from build123d import *

# Parameters (mm, degrees)
F0_W     = 600
F0_H     = 200
F1_DEPTH = 290
F2_R     = 50
F3_T     = -2


with BuildPart() as f1:
    # F0 (on Front) → F1 (new body)
    with BuildSketch(Plane.XZ):
        with Locations((300, 100)):
            Rectangle(F0_W, F0_H)
    extrude(amount=F1_DEPTH)

    # F2
    f2_edges = [f1.edges().sort_by_distance(p)[0] for p in [
        (600, -290, 100),
        (0, -290, 100),
        (600, 0, 100),
        (600, -145, 0),
        (300, -290, 0),
        (0, -145, 0),
        (0, 0, 100),
        (300, 0, 0),
    ]]
    fillet(f2_edges, radius=F2_R)

    # F3
    f3_openings = [f1.faces().sort_by_distance(p)[0] for p in [
        (300, -145, 200),
    ]]
    offset(amount=F3_T, openings=f3_openings)


solid = f1.part
Source: CAD feature listing. Evaluate the final solid. Frame: model axes, mm. A direction names the side the tool comes from. Give positions to 0.01 mm unless a question says otherwise; leave off trailing zeros. Order: outer loops, then holes, each group sorted by start corner. A loop starts at its lowest first (then second) coordinate and runs counter-clockwise, first axis right, second up. Notation, with made-up numbers: (-5, 78.5) -> (33, 78.5) arc R22 ccw to (33, 84.5) -> close; hole circle Ø3 at (35, -23). An arc over 180 degrees is marked (long way). Use a Markdown table: item, result.
1) Contact query for flat-ended pins moving along their axis: P1, Ø5, axis at x = 500.5, y = -116, coming from the +Z side; P2, Ø8, axis at y = -260.5, z = 154, coming from the -X side. Output: stop coordinate, or through.
Answer list:
| item | result |
|---|---|
| P1 | z = 2 |
| P2 | x = 2.8 |
2) Section query C-C, the plane x = 82. Return the cut outline in (y, z), then the cut area to 3 significant figures.
Answer list:
| item | result |
|---|---|
| outline | (-290, 50) arc R50 ccw to (-240, 0) -> (-50, 0) arc R50 ccw to (0, 50) -> (0, 200) -> (-2, 200) -> (-2, 50) arc R48 cw to (-50, 2) -> (-240, 2) arc R48 cw to (-288, 50) -> (-288, 200) -> (-290, 200) -> close |
| area | 1,290 mm² |
3) Section query A-A, the plane z = 114. Return the cut outline in (x, y).
Answer list:
| item | result |
|---|---|
| outline | (0, -240) arc R50 ccw to (50, -290) -> (550, -290) arc R50 ccw to (600, -240) -> (600, -50) arc R50 ccw to (550, 0) -> (50, 0) arc R50 ccw to (0, -50) -> close; hole (2, -240) arc R48 ccw to (50, -288) -> (550, -288) arc R48 ccw to (598, -240) -> (598, -50) arc R48 ccw to (550, -2) -> (50, -2) arc R48 ccw to (2, -50) -> close |
4) Ray query, line 1 along Y through (x, z) = (219.5, 85); line 2 along X through (y, z) = (-61, 99); line 3 along Y through (x, z) = (71, 38.5). Return the intervals inside material, ascending. Write a range as [from, to].
Answer list:
| item | result |
|---|---|
| line 1 | [-290, -288], [-2, 0] |
| line 2 | [0, 2], [598, 600] |
| line 3 | [-288.66, -286.6], [-3.4, -1.34] |
5) Section query B-B, the plane y = -138. Return the cut outline in (x, z), then the cut area to 3 significant figures.
Answer list:
| item | result |
|---|---|
| outline | (0, 50) arc R50 ccw to (50, 0) -> (550, 0) arc R50 ccw to (600, 50) -> (600, 200) -> (598, 200) -> (598, 50) arc R48 cw to (550, 2) -> (50, 2) arc R48 cw to (2, 50) -> (2, 200) -> (0, 200) -> close |
| area | 1,910 mm² |
6) Section query D-D, the plane z = 41. Return the cut outline in (x, y).
Answer list:
| item | result |
|---|---|
| outline | (0.82, -240) arc R49.18 ccw to (50, -289.18) -> (550, -289.18) arc R49.18 ccw to (599.18, -240) -> (599.18, -50) arc R49.18 ccw to (550, -0.82) -> (50, -0.82) arc R49.18 ccw to (0.82, -50) -> close; hole (2.85, -240) arc R47.15 ccw to (50, -287.15) -> (550, -287.15) arc R47.15 ccw to (597.15, -240) -> (597.15, -50) arc R47.15 ccw to (550, -2.85) -> (50, -2.85) arc R47.15 ccw to (2.85, -50) -> close |
7) Mould query, pull axis Y, two halves, no side actions, for faces 3 (the cylindrical face through (303.5, -15.036, 14.258)), 4 (the flat face through (598, -144, 124)), 5 (the flat face through (0, -144, 124)). Classes: +Y half, -Y half, draft (parallel to the pull), parting line (faces both ways), or undercut.
Answer list:
| item | result |
|---|---|
| face 3 | +Y half |
| face 4 | undercut |
| face 5 | draft |
8) Reachability of faces 1 (the cylindrical face through (14.258, -274.964, 126.05)), 2 (the cylindrical face through (15.69, -273.57, 126.05)) from +Z, -Z, +X, -X, +Y, -Y: full face, straight path, thin tool, end or side. Return the list, or none.
Answer list:
| item | result |
|---|---|
| face 1 | +Z, -Z, -X, -Y |
| face 2 | +Z |
